Autodesk Inventor part; units mm, degrees
ref_plane "YZ Plane" through (0, 0, 0) normal (1, 0, 0) x (0, 1, 0)
ref_plane "XZ Plane" through (0, 0, 0) normal (0, 1, 0) x (-1, 0, 0)
ref_plane "XY Plane" through (0, 0, 0) normal (0, 0, 1) x (1, 0, 0)
sketch "Esquisse1" plane through (0, 0, 0) normal (1, 0, 0) x (0, 1, 0)
  line L0 (95, 10) -> (-95, 10)
  line L1 (-95, 10) -> (-95, -10)
  line L2 (-95, -10) -> (95, -10)
  line L3 (95, -10) -> (95, 10)
  line L4 (95, 10) -> (-95, -10)
  line L5 (-95, 10) -> (95, -10)
  point P0 (0, 0)
  point P1 (0, 0)
  point P2 (0, 0)
  dimension "d0" = 190
  dimension "d1" = 20
extrude "Extrusion1" add sketch "Esquisse1" along normal blind 20
sketch "Esquisse2" plane through (0, 95, 10) normal (0, 1, 0) x (1, 0, 0)
  line L0 (20, 20) -> (20, 0)
  line L1 (0, 0) -> (20, 0)
  line L2 (20, 0) -> (20, 4)
  line L3 (20, 4) -> (0, 4)
  line L4 (0, 4) -> (0, 0)
  line L5 (0, 10) -> (20, 10)
  line L6 (0, 20) -> (20, 20)
  line L7 (20, 20) -> (20, 16)
  line L8 (20, 16) -> (0, 16)
  line L9 (0, 16) -> (0, 20)
extrude "Extrusion2" add sketch "Esquisse2" along normal blind 20
sketch "Esquisse3" plane through (0, -95, 10) normal (0, 0, 1) x (1, 0, 0)
  circle A0 centre (10, 200) radius 1.765
  line L0 (0, 0) -> (0, 210)
  line L1 (0, 210) -> (20, 210)
  point P0 (0, 95)
  dimension "d6" = 3.53
  dimension "d7" = 10
  dimension "d8" = 10
extrude "Extrusion3" cut sketch "Esquisse3" against normal blind 78.75
sketch "Esquisse4" plane through (0, -95, 10) normal (0, 0, 1) x (1, 0, 0)
  line L0 (20, 190) -> (0, 190)
  line L1 (5, 0) -> (15, 0)
  line L2 (15, 0) -> (15, 190)
  line L3 (15, 190) -> (5, 190)
  line L4 (5, 190) -> (5, 0)
  point P0 (0, 95)
extrude "Extrusion4" cut sketch "Esquisse4" against normal blind 5
sketch "Esquisse5" plane through (20, -95, -10) normal (0, 0, -1) x (-1, 0, 0)
  line L0 (5, 0) -> (0, 0)
  line L1 (15, 0) -> (15, 190)
  line L2 (5, 0) -> (15, 0)
  line L3 (15, 0) -> (15, 190)
  line L4 (15, 190) -> (5, 190)
  line L5 (5, 190) -> (5, 0)
  point P0 (20, 95)
extrude "Extrusion5" cut sketch "Esquisse5" against normal blind 5
sketch "Esquisse6" plane through (20, 0, 0) normal (1, 0, 0) x (0, 0, -1)
  line L0 (-10, -95) -> (10, -95)
  line L1 (5, -95) -> (5, 95)
  line L2 (-5, -95) -> (5, -95)
  line L3 (5, -95) -> (5, 88)
  line L4 (5, 88) -> (-5, 88)
  line L5 (-5, 88) -> (-5, -95)
  point P0 (0, 0)
extrude "Extrusion6" cut sketch "Esquisse6" against normal blind 5
sketch "Esquisse7" plane through (0, 0, 0) normal (-1, 0, 0) x (0, 0, 1)
  line L0 (-5, 88) -> (-5, -95)
  line L1 (5, -95) -> (5, 95)
  line L2 (-5, -95) -> (5, -95)
  line L3 (5, -95) -> (5, 88)
  line L4 (5, 88) -> (-5, 88)
  line L5 (-5, 88) -> (-5, -95)
  point P0 (0, 0)
extrude "Extrusion7" cut sketch "Esquisse7" against normal blind 5
properties part number "rail_principal"
Check sheet for the modelled part. Datum: model origin and axes. Units: mm. A direction names the side the tool comes from. Coordinates: 2 decimals unless noted, no trailing zeros. Loops run counter-clockwise (first coordinate to the right, second up) from the corner with the lowest first, then second, coordinate; pieces in that order, holes last. Notation, with made-up numbers: (15, 72) -> (22, 72) arc R31 cw to (22, 111) -> close; hole circle Ø6 at (-26.5, 33.25). An arc over 180 degrees is marked (long way). Answer in a Markdown table with one row per item.
1. Material ranges on line 1 along Z through (x, y) = (2, 15); line 2 along Y through (x, z) = (10, 9.1) (3 decimals); line 3 along X through (y, z) = (54, -6), recorded low to high. Write a range as [from, to].
Check values:
| item | result |
|---|---|
| line 1 | z = [-10, -5], [5, 10] |
| line 2 | y = [95, 103.235], [106.765, 115] |
| line 3 | x = [0, 5], [15, 20] |
2. Access from +Z, -Z, +X, -X, +Y, -Y to the whole of each face (thin tool, end or side, straight path). Record for faces 1 (the face through (18, 88, 0)), 2 (the face through (2, 88, 0)), 3 (the face through (10, 103, 6)).
Check values:
| item | result |
|---|---|
| face 1 | +X, -Y |
| face 2 | -X, -Y |
| face 3 | +X, -X, +Y |
3. Release check for a two-part mould opening along Z. For faces 4 (the face through (10, 103, -6)), 5 (the face through (15, 1, -8)), 6 (the face through (3, 9, -10)) record: released by +Z, released by -Z, zero draft, split by the parting line, or undercut.
Check values:
| item | result |
|---|---|
| face 4 | undercut |
| face 5 | zero draft |
| face 6 | released by -Z |
4. Sectioned sample at A-A, the plane y = 105. Record the boundary of the cut face in (x, z) (3 decimals).
Check values:
| item | result |
|---|---|
| outline | (0, -10) -> (8.235, -10) -> (8.235, -6) -> (0, -6) -> close; (0, 6) -> (8.235, 6) -> (8.235, 10) -> (0, 10) -> close; (11.765, -10) -> (20, -10) -> (20, -6) -> (11.765, -6) -> close; (11.765, 6) -> (20, 6) -> (20, 10) -> (11.765, 10) -> close |
5. Sectioned sample at B-B, the plane x = 10. Record the boundary of the cut face in (y, z) (3 decimals), then the cut area to 3 significant figures.
Check values:
| item | result |
|---|---|
| outline | (-95, -5) -> (95, -5) -> (95, 5) -> (-95, 5) -> close; (95, -10) -> (103.235, -10) -> (103.235, -6) -> (95, -6) -> close; (95, 6) -> (103.235, 6) -> (103.235, 10) -> (95, 10) -> close; (106.765, -10) -> (115, -10) -> (115, -6) -> (106.765, -6) -> close; (106.765, 6) -> (115, 6) -> (115, 10) -> (106.765, 10) -> close |
| area | 2,030 mm2 |
6. Sectioned sample at D-D, the plane z = -0.5. Record the boundary of the cut face in (x, y).
Check values:
| item | result |
|---|---|
| outline | (0, 88) -> (5, 88) -> (5, -95) -> (15, -95) -> (15, 88) -> (20, 88) -> (20, 95) -> (0, 95) -> close |
7. Go/stop test with flat-tipped pins: pin 1 (1 mm diameter, centred on y = -31.5, z = 2.5, fed in from -X); pin 2 (4.5 mm diameter, centred on x = 11.5, z = -7.5, fed in from -Y); pin 3 (2.5 mm diameter, centred on x = 17.5, z = 1.5, fed in from -Y). Record where each tip stops, or that it passes through.
Check values:
| item | result |
|---|---|
| pin 1 | stops at x = 5 |
| pin 2 | stops at y = 95 |
| pin 3 | stops at y = 88 |
